```python
from build123d import *
from build123d import SkipClean  # not in build123d's __all__

# Parameters (mm, degrees)
F0_R     = 8.89
F0_R_2   = 5.969
F3_R     = 7.62
F3_R_2   = 5.969
F4_R     = 7.62
F4_R_2   = 5.969
F5_DEPTH = 25.4


with BuildPart() as f2:
    # F2: sweep along a path in F1
    with BuildLine(Plane.XY) as f2_path:
        Line((0, 0), (0, 33.02))
        ThreePointArc((0, 33.02), (13.97, 46.99), (27.94, 33.02))
        Line((27.94, 33.02), (27.94, 0))
    # F0 (on Front) → F2 (sweep)
    with BuildSketch(Plane.XZ):
        Circle(F0_R)
        Circle(F0_R_2, mode=Mode.SUBTRACT)
    sweep(path=f2_path.line)

    # F3 (on face) + F4 (on face) → F5 (join)
    with BuildSketch(Plane.XZ):
        Circle(F3_R)
        Circle(F3_R_2, mode=Mode.SUBTRACT)
    with BuildSketch(Plane.XZ):
        with Locations((27.94, 0)):
            Circle(F4_R)
        with Locations((27.94, 0)):
            Circle(F4_R_2, mode=Mode.SUBTRACT)
    with SkipClean():  # cleaning this boolean's faces spoils the solid; the shape is the same uncleaned
        extrude(amount=F5_DEPTH)


solid = f2.part
```
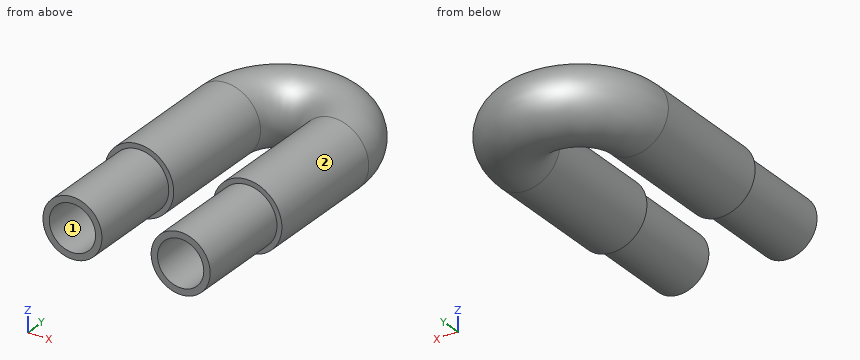
Geometry: final body of the model. Coordinates: model frame, mm. Face numbers are marked on the shaded views. Coordinates: 2 decimals unless noted, no trailing zeros. Order: outer loops, then holes, each group sorted by start corner. A loop starts at its lowest first (then second) coordinate and runs counter-clockwise, first axis right, second up. Notation, with made-up numbers: (30.25, 56.25) - (56.25, 56.25) arc R26 ccw to (56.25, 95.25) - close; hole circle Ø1 at (63.25, 2.25). An arc over 180 degrees is marked (long way). Write each question's results on one line, items separated by ' | '.
(1) Section query A-A, the plane y = 11. Return the cut outline in (x, z), plus the area to 3 significant figures.
Values found:
outline: circle Ø17.78 at (0, 0); circle Ø17.78 at (27.94, 0); hole circle Ø11.94 at (0, 0); hole circle Ø11.94 at (27.94, 0) | area: 273 mm²
(2) Section query B-B, the plane z = 0. Return the cut outline in (x, y), plus the area to 3 significant figures.
Values found:
outline: (-8.89, 0) - (-7.62, 0) - (-7.62, -25.4) - (-5.97, -25.4) - (-5.97, 33.02) arc R19.94 cw to (33.91, 33.02) - (33.91, -25.4) - (35.56, -25.4) - (35.56, 0) - (36.83, 0) - (36.83, 33.02) arc R22.86 ccw to (-8.89, 33.02) - close; (5.97, -25.4) - (7.62, -25.4) - (7.62, 0) - (8.89, 0) - (8.89, 33.02) arc R5.08 cw to (19.05, 33.02) - (19.05, 0) - (20.32, 0) - (20.32, -25.4) - (21.97, -25.4) - (21.97, 33.02) arc R8 ccw to (5.97, 33.02) - close | area: 810 mm²
(3) Mould query, pull axis X, two halves, no side actions, for the marked faces 1 and 2. Classes: +X half, -X half, draft (parallel to the pull), parting line (faces both ways), or undercut.
Values found:
face 1: undercut | face 2: undercut
(4) Line query: line 1 (X direction, y = 22, z = 0); line 2 (Z direction, x = 27.94, y = 12.5); line 3 (X direction, y = 31.5, z = 3.5). Output: solid intervals per line, ascending. Write a range as [from, to].
Values found:
line 1: x = [-8.89, -5.97], [5.97, 8.89], [19.05, 21.97], [33.91, 36.83] | line 2: z = [-8.89, -5.97], [5.97, 8.89] | line 3: x = [-8.17, -4.84], [4.84, 8.17], [19.77, 23.1], [32.78, 36.11]
(5) Section query C-C, the plane z = 4. Return the cut outline in (x, y).
Values found:
outline: (-7.94, 0) - (-6.49, 0) - (-6.49, -25.4) - (-4.43, -25.4) - (-4.43, 33.02) arc R18.4 cw to (32.37, 33.02) - (32.37, -25.4) - (34.43, -25.4) - (34.43, 0) - (35.88, 0) - (35.88, 33.02) arc R21.91 ccw to (-7.94, 33.02) - close; (4.43, -25.4) - (6.49, -25.4) - (6.49, 0) - (7.94, 0) - (7.94, 33.02) arc R6.03 cw to (20, 33.02) - (20, 0) - (21.45, 0) - (21.45, -25.4) - (23.51, -25.4) - (23.51, 33.02) arc R9.54 ccw to (4.43, 33.02) - close
(6) First-contact query: pin 1 Ø7 at (x, z) = (27.94, 0) entering from -Y; pin 2 Ø6 at (x, y) = (12, 29) entering from +Z; pin 3 Ø1.5 at (x, z) = (17, -0.5) entering from -Y; pin 4 Ø12 at (x, y) = (16.5, -9.5) entering from -Z. Flat tips, straight axial feed; report the tip coordinate or a pass-through.
Values found:
pin 1: stops at y = 42.63 | pin 2: passes through | pin 3: stops at y = 36.43 | pin 4: stops at z = -5.34
(7) Section query D-D, the plane y = -10. Return the cut outline in (x, z).
Values found:
outline: circle Ø15.24 at (0, 0); circle Ø15.24 at (27.94, 0); hole circle Ø11.94 at (0, 0); hole circle Ø11.94 at (27.94, 0)
